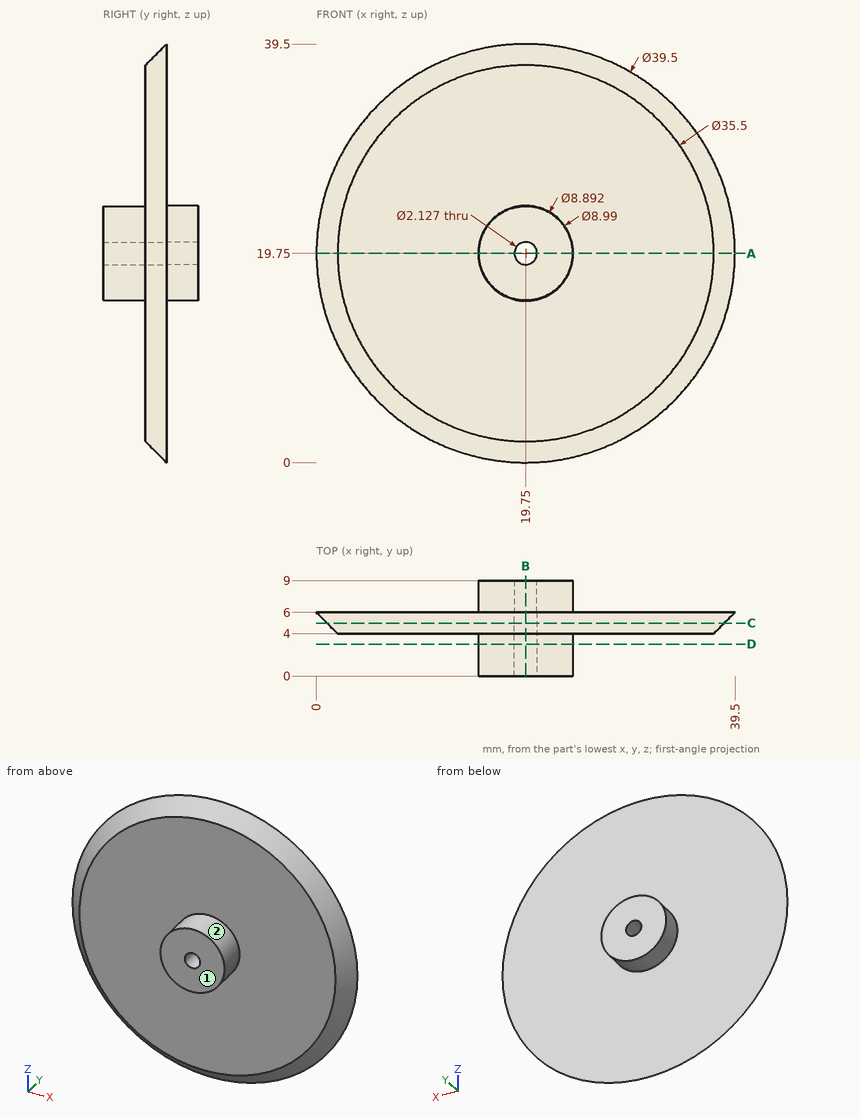
Here's the drawing with two shaded views (mm, measured from the low corner). I have some questions. A direction names the side the tool comes from. Coordinates: 2 decimals unless noted, no trailing zeros. Order: outer loops, then holes, each group sorted by start corner. A loop starts at its lowest first (then second) coordinate and runs counter-clockwise, first axis right, second up. Notation, with made-up numbers: (43.5, 87.25) - (52.5, 87.25) arc R22 ccw to (52.5, 94.25) - close; hole circle Ø6 at (86, -32.75). An arc over 180 degrees is marked (long way). Answer in a Markdown table with one row per item.
1. For the marked faces 1 and 2, which set-ups out of +Z, -Z, +X, -X, +Y, -Y let a thin tool reach every point of the face, with its end or its side?
Reply:
| item | result |
|---|---|
| face 1 | +Z, -Z, +X, -X, -Y |
| face 2 | -Y |
2. Suppose I cut it at A-A (z = 19.75). Please give me the cut outline in (x, y) (1 decimal).
Reply:
| item | result |
|---|---|
| outline | (0, 6) - (2, 4) - (15.3, 4) - (15.3, 0) - (18.7, 0) - (18.7, 9) - (15.3, 9) - (15.3, 6) - close; (20.8, 0) - (24.2, 0) - (24.2, 4) - (37.5, 4) - (39.5, 6) - (24.2, 6) - (24.2, 9) - (20.8, 9) - close |
3. For pin 1 (12 mm diameter, centred on x = 11.5, z = 7.5, fed in from +Y); pin 2 (1.5 mm diameter, centred on y = 2, z = 18, fed in from +X); pin 3 (3 mm diameter, centred on x = 25, y = 2, fed in from +Z), each with a flat end and sliding along its axis, tell me the tip position at first contact or that it passes through.
Reply:
| item | result |
|---|---|
| pin 1 | stops at y = 6 |
| pin 2 | stops at x = 24.08 |
| pin 3 | stops at z = 22.14 |
4. If I drill on line 1 along Z through (x, y) = (19.75, 8.35) (1 decimal); line 2 along Y through (x, z) = (17, 14.5); line 3 along Z through (x, y) = (19.75, 4.45), over which ranges is the centre line in solid material (lowest first)?
Reply:
| item | result |
|---|---|
| line 1 | z = 15.3 to 18.7, 20.8 to 24.2 |
| line 2 | y = 4 to 6 |
| line 3 | z = 1.55 to 18.69, 20.81 to 37.95 |
5. Suppose I cut it at C-C (y = 5). Please give me the cut outline in (x, z), and give its area (3 significant figures).
Reply:
| item | result |
|---|---|
| outline | circle Ø37.5 at (19.75, 19.75); hole circle Ø2.13 at (19.75, 19.75) |
| area | 1,100 mm^2 |
6. Suppose I cut it at B-B (x = 19.75). Please give me the cut outline in (y, z) (1 decimal).
Reply:
| item | result |
|---|---|
| outline | (0, 15.3) - (4, 15.3) - (4, 2) - (6, 0) - (6, 15.3) - (9, 15.3) - (9, 18.7) - (0, 18.7) - close; (0, 20.8) - (9, 20.8) - (9, 24.2) - (6, 24.2) - (6, 39.5) - (4, 37.5) - (4, 24.2) - (0, 24.2) - close |
7. Suppose I cut it at D-D (y = 3). Please give me the cut outline in (x, z).
Reply:
| item | result |
|---|---|
| outline | circle Ø8.89 at (19.75, 19.75); hole circle Ø2.13 at (19.75, 19.75) |
